Here's how the part is built. I have some questions about the finished solid (model axes, mm). Face numbers are marked on the shaded views. A direction names the side the tool comes from. Coordinates: 2 decimals unless noted, no trailing zeros. Write each loop counter-clockwise with the first axis right and the second up, starting at its lowest first coordinate (ties: lowest second). Pieces come first, ordered by that corner, then holes.
(1) Imagine slicing it at D-D, the plane x = 7. List the corners of the cut face in (y, z) for me.
(2) Please list where these lines run through material, in increasing order: probe 1 along Y at (x, z) = (0, -30); probe 2 along X at (y, z) = (-6.5, -30.05); probe 3 along X at (y, z) = (0.5, -29.7).
(3) Thinking about a two-plate mould opening in X: for the marked faces 6, 7 and 8, which applies, released by +X, released by -X, zero draft, split by the parting line, or undercut?
(4) Imagine slicing it at A-A, the plane x = 0. List the corners of the cut face in (y, z) for me, plus the area to 3 significant figures.
(5) Which directions (+Z, -Z, +X, -X, +Y, -Y) give clear straight access to the entire face, cutting with the end or side of a thin tool? Please do the marked faces 1, 2, 3, 4 and 5.
(6) For pin 1 Ø6.5 at (x, y) = (0, 0) entering from +Z; pin 2 Ø0.6 at (x, z) = (0, -30.5) entering from -Y; pin 3 Ø1 at (x, z) = (10.5, -30.5) entering from -Y; pin 4 Ø1 at (y, z) = (11, -30.5) entering from -X, each with a flat end and sliding along its axis, tell me the tip position at first contact or that it passes through.
```python
from build123d import *

# Parameters (mm, degrees)
SKETCH005_R           = 12
PAD002_DEPTH          = 2
SKETCH004_W           = 2.57
SKETCH004_H           = 3.2
POCKET003_DEPTH       = 5
POLARPATTERN001_COUNT = 8
SKETCH006_R           = 2
POCKET002_DEPTH       = 6
FILLET001_R           = 1


with BuildPart() as part:
    # Sketch005 → Pad002 (new body)
    with BuildSketch(Plane.XY.offset(28.5)):
        Circle(SKETCH005_R)
    extrude(amount=PAD002_DEPTH)

    # Sketch004 (on Face3 of Pad002) → Pocket003 (cut)
    with BuildSketch(Plane.XY.offset(30.5)):
        with Locations((11.125, 0)):
            Rectangle(SKETCH004_W, SKETCH004_H)
    pocket003 = extrude(amount=-POCKET003_DEPTH, mode=Mode.SUBTRACT)

    # PolarPattern001: Pocket003 ×8 about axis
    polarpattern001_axis = Axis((0, 0, 30.5), (0, 0, 1))
    for i in range(1, POLARPATTERN001_COUNT):
        add(pocket003.rotate(polarpattern001_axis, i * 360 / POLARPATTERN001_COUNT), mode=Mode.SUBTRACT)

    # Sketch006 (on Face4 of PolarPattern001) → Pocket002 (cut)
    with BuildSketch(Plane.XY.offset(30.5)):
        Circle(SKETCH006_R)
    extrude(amount=-POCKET002_DEPTH, mode=Mode.SUBTRACT)

    # Fillet001
    fillet001_edges = [part.edges().sort_by_distance(p)[0] for p in [
        (-2, 0, 28.5),
    ]]
    fillet(fillet001_edges, radius=FILLET001_R)


with BuildPart() as part_1:
    # Body002 placement: moved
    add(part.part.moved(Location((0, 0, -60))))


solid = part_1.part
```
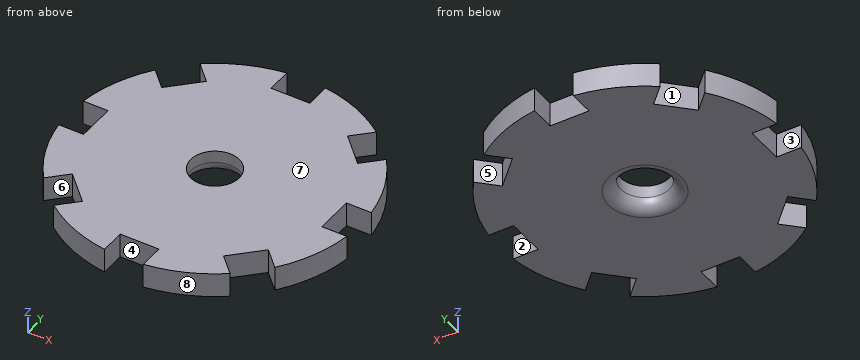
Recorded:
1. outline: (-9.75, -31.5) - (-9.26, -31.5) - (-9.26, -29.5) - (-9.75, -29.5) - close; (-6.92, -31.5) - (6.92, -31.5) - (6.92, -29.5) - (-6.92, -29.5) - close; (9.26, -31.5) - (9.75, -31.5) - (9.75, -29.5) - (9.26, -29.5) - close
2. probe 1: y = -9.84 to -2, 2 to 9.84
2. probe 2: x = -10.09 to -8.76, -7.42 to 7.42, 8.76 to 10.09
2. probe 3: x = -9.84 to -1.94, 1.94 to 9.84
3. face 6: undercut
3. face 7: zero draft
3. face 8: released by +X
4. outline: (-9.84, -31.5) - (-3, -31.5) arc R1 ccw to (-2, -30.5) - (-2, -29.5) - (-9.84, -29.5) - close; (2, -30.5) arc R1 ccw to (3, -31.5) - (9.84, -31.5) - (9.84, -29.5) - (2, -29.5) - close
4. area: 30.9 mm2
5. face 1: +Z, -Z
5. face 2: +Z, -Z, +X
5. face 3: +Z, -Z, -X
5. face 4: +Z, -Z, -Y
5. face 5: +Z, -Z, +Y
6. pin 1: stops at z = -29.5
6. pin 2: stops at y = -9.84
6. pin 3: stops at y = -6.63
6. pin 4: stops at x = -5.81
